from build123d import *

# Parameters (mm, degrees)
SKETCH1_W           = 259
SKETCH1_H           = 25
BOSS_EXTRUDE1_DEPTH = 5
SKETCH4_W           = 29
SKETCH4_H           = 5.3
CUT_EXTRUDE2_DEPTH  = 6
SKETCH5_R           = 1.65
CUT_EXTRUDE3_DEPTH  = 6
SKETCH6_R           = 1.65
CUT_EXTRUDE4_DEPTH  = 6
FILLET1_R           = 5


with BuildPart() as part:
    # Sketch1 → Boss-Extrude1 (new body)
    with BuildSketch(Plane(origin=(0, 0, 0), x_dir=(1, 0, 0), z_dir=(0, 1, 0))):
        with Locations((129.5, 12.5)):
            Rectangle(SKETCH1_W, SKETCH1_H)
    extrude(amount=BOSS_EXTRUDE1_DEPTH)

    # Sketch4 → Cut-Extrude2 (cut, through all)
    with BuildSketch(Plane(origin=(0, 5, 0), x_dir=(1, 0, 0), z_dir=(0, 1, 0))):
        with Locations((43.05, 12.5)):
            Rectangle(SKETCH4_W, SKETCH4_H)
        with Locations((100.45, 12.5)):
            Rectangle(SKETCH4_W, SKETCH4_H)
        with Locations((157.85, 12.5)):
            Rectangle(SKETCH4_W, SKETCH4_H)
        with Locations((215.25, 12.5)):
            Rectangle(SKETCH4_W, SKETCH4_H)
    extrude(amount=-CUT_EXTRUDE2_DEPTH, mode=Mode.SUBTRACT)

    # Sketch5 → Cut-Extrude3 (cut, through all)
    with BuildSketch(Plane(origin=(0, 5, 0), x_dir=(1, 0, 0), z_dir=(0, 1, 0))):
        with Locations((28.55, 15.15)):
            Circle(SKETCH5_R)
        with Locations((28.55, 9.85)):
            Circle(SKETCH5_R)
        with Locations((57.55, 15.15)):
            Circle(SKETCH5_R)
        with Locations((57.55, 9.85)):
            Circle(SKETCH5_R)
        with Locations((85.95, 15.15)):
            Circle(SKETCH5_R)
        with Locations((85.95, 9.85)):
            Circle(SKETCH5_R)
        with Locations((114.95, 15.15)):
            Circle(SKETCH5_R)
        with Locations((114.95, 9.85)):
            Circle(SKETCH5_R)
        with Locations((143.35, 15.15)):
            Circle(SKETCH5_R)
        with Locations((143.35, 9.85)):
            Circle(SKETCH5_R)
        with Locations((172.35, 15.15)):
            Circle(SKETCH5_R)
        with Locations((172.35, 9.85)):
            Circle(SKETCH5_R)
        with Locations((200.75, 15.15)):
            Circle(SKETCH5_R)
        with Locations((229.75, 15.15)):
            Circle(SKETCH5_R)
        with Locations((229.75, 9.85)):
            Circle(SKETCH5_R)
        with Locations((200.75, 9.85)):
            Circle(SKETCH5_R)
    extrude(amount=-CUT_EXTRUDE3_DEPTH, mode=Mode.SUBTRACT)

    # Sketch6 → Cut-Extrude4 (cut, through all)
    with BuildSketch(Plane.XZ):
        with Locations((193.4, -21.5)):
            Circle(SKETCH6_R)
        with Locations((176.6, -21.5)):
            Circle(SKETCH6_R)
        with Locations((159.8, -21.5)):
            Circle(SKETCH6_R)
        with Locations((143, -21.5)):
            Circle(SKETCH6_R)
        with Locations((126.2, -21.5)):
            Circle(SKETCH6_R)
        with Locations((109.4, -21.5)):
            Circle(SKETCH6_R)
        with Locations((92.6, -21.5)):
            Circle(SKETCH6_R)
        with Locations((75.8, -21.5)):
            Circle(SKETCH6_R)
        with Locations((59, -21.5)):
            Circle(SKETCH6_R)
    extrude(amount=-CUT_EXTRUDE4_DEPTH, mode=Mode.SUBTRACT)

    # Fillet1
    fillet1_edges = [part.edges().sort_by_distance(p)[0] for p in [
        (259, 2.5, -25),
        (259, 2.5, 0),
    ]]
    fillet(fillet1_edges, radius=FILLET1_R)


solid = part.part
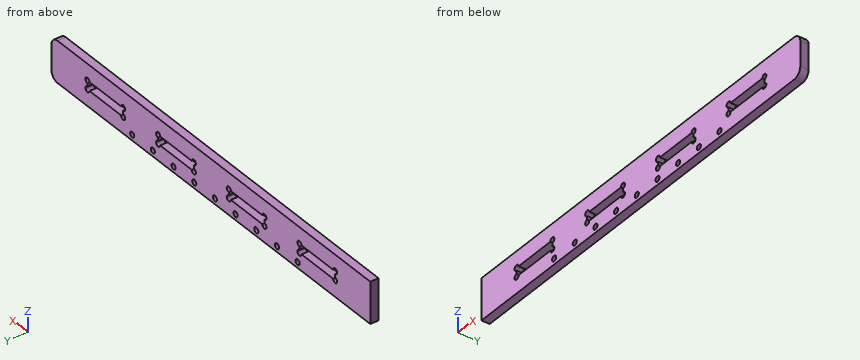
CAD build for the part. Positions are in the model's coordinates, mm. Round coordinates to 2 decimals unless told otherwise and drop trailing zeros. Loops run counter-clockwise (first coordinate to the right, second up) from the corner with the lowest first, then second, coordinate; pieces in that order, holes last. Notation, with made-up numbers: (77, -33.75) - (106, -33.75) arc R7 ccw to (106, -23.75) - close; hole circle Ø3 at (69, 14). An arc over 180 degrees is marked (long way). Put each result on its own line as item: value.
1. Slice it at B-B on y = 3.75. Give the number of separate pieces and of enclosed holes in the cut face, and give its area (3 significant figures).
Geometry check:
separate pieces: 1
enclosed holes: 13
area: 5,670 mm²
2. Pin check, flat tips, straight feed: P1, Ø2, axis at y = 3.5, z = -22.5, coming from the +X side; P2, Ø2.5, axis at x = 172.35, z = -9.85, coming from the -Y side. Stop position of each tip, or through.
Geometry check:
P1: x = 258.77
P2: through
3. Slice it at A-A on x = 100. List the corners of the cut face in (y, z), and give its area (3 significant figures).
Geometry check:
outline: (0, -25) - (5, -25) - (5, -15.15) - (0, -15.15) - close; (0, -9.85) - (5, -9.85) - (5, 0) - (0, 0) - close
area: 98.5 mm²
4. Wall check: line 1 (Z direction, x = 92.6, y = 1.5); line 2 (X direction, y = 3.15, z = -11.75); line 3 (Z direction, x = 86, y = 1.4). Give the ranges that are in metal, low to high.
Geometry check:
line 1: -25 to -23.15, -19.85 to -15.15, -9.85 to 0
line 2: 0 to 28.55, 57.55 to 85.95, 114.95 to 143.35, 172.35 to 200.75, 229.75 to 259
line 3: -25 to -16.8, -8.2 to 0
